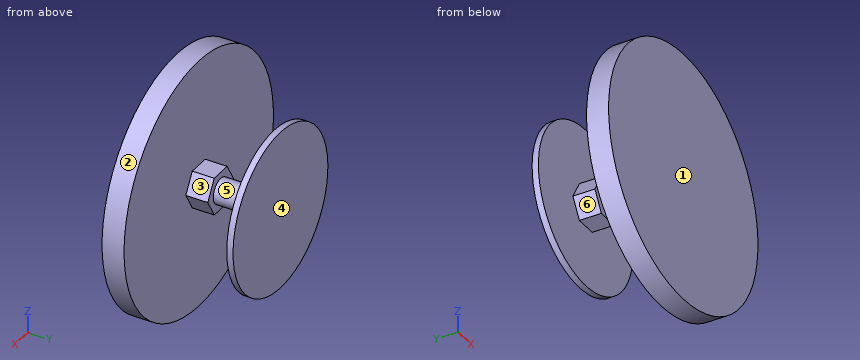
from build123d import *

# Parameters (mm, degrees)
ESBO_O2_R                = 40
RESSALTO_EXTRUS_O1_DEPTH = 7
RESSALTO_EXTRUS_O2_DEPTH = 7
ESBO_O4_R                = 4
RESSALTO_EXTRUS_O3_DEPTH = 10
RESSALTO_EXTRUS_O4_DEPTH = 7
ESBO_O6_R                = 25.4
RESSALTO_EXTRUS_O5_DEPTH = 2


with BuildPart() as part:
    # Esboço2 → Ressalto-extrusão1 (new body)
    with BuildSketch(Plane(origin=(0, 0, 0), x_dir=(1, 0, 0), z_dir=(0, 1, 0))):
        with Locations(Location((0, 0, 0), (0, 0, 270))):
            Circle(ESBO_O2_R)
    extrude(amount=RESSALTO_EXTRUS_O1_DEPTH)

    # Esboço3 → Ressalto-extrusão2 (add)
    with BuildSketch(Plane(origin=(0, 7, 0), x_dir=(1, 0, 0), z_dir=(0, 1, 0))):
        Polygon((6.92820323, 0), (3.464101615, 6), (-3.464101615, 6), (-6.92820323, 0), (-3.464101615, -6), (3.464101615, -6), align=None)
    extrude(amount=RESSALTO_EXTRUS_O2_DEPTH)

    # Esboço4 → Ressalto-extrusão3 (add)
    with BuildSketch(Plane(origin=(0, 14, 0), x_dir=(1, 0, 0), z_dir=(0, 1, 0))):
        with Locations(Location((0, 0, 0), (0, 0, 270))):
            Circle(ESBO_O4_R)
    extrude(amount=RESSALTO_EXTRUS_O3_DEPTH)

    # Esboço5 → Ressalto-extrusão4 (add)
    with BuildSketch(Plane(origin=(0, 24, 0), x_dir=(1, 0, 0), z_dir=(0, 1, 0))):
        Polygon((6.92820323, 0), (3.464101615, 6), (-3.464101615, 6), (-6.92820323, 0), (-3.464101615, -6), (3.464101615, -6), align=None)
    extrude(amount=RESSALTO_EXTRUS_O4_DEPTH)

    # Esboço6 → Ressalto-extrusão5 (add)
    with BuildSketch(Plane(origin=(0, 31, 0), x_dir=(1, 0, 0), z_dir=(0, 1, 0))):
        with Locations(Location((0, 0, 0), (0, 0, 270))):
            Circle(ESBO_O6_R)
    extrude(amount=RESSALTO_EXTRUS_O5_DEPTH)


solid = part.part
Read the model definition and answer for the solid it produces. Units are mm, in the model's axes. Face numbers are marked on the shaded views. A direction names the side the tool comes from. Round coordinates to 2 decimals unless told otherwise and drop trailing zeros. Order: outer loops, then holes, each group sorted by start corner. A loop starts at its lowest first (then second) coordinate and runs counter-clockwise, first axis right, second up. Notation, with made-up numbers: (-4, -34) - (53, -34) arc R34 cw to (53, -3) - close; hole circle Ø7 at (-16, 50). An arc over 180 degrees is marked (long way). Use one line per item in the form item = value. Start each with the question number.
(1) Find the intervals of material crossed by line 1 along Y through (x, z) = (-16.5, 18); line 2 along Y through (x, z) = (33.5, 8.5); line 3 along Z through (x, y) = (-2, 20.5), in increasing order. Write a range as from..to.
(2) The part is cut by section D-D (y = 10). Give the vertices of the cut face in (x, z).
(3) For the marked faces 4, 5 and 6, determine the directions among +Z, -Z, +X, -X, +Y, -Y from which every point of the face is accessible in a straight line to the end or side of a thin tool.
(4) Determine the mould class of the marked faces 1, 2 and 3 for opening direction Y: +Y half, -Y half, draft (parallel to the pull), parting line (faces both ways), or undercut.
(5) The part is cut by section A-A (x = 20.5). Give the vertices of the cut face in (y, z).
(6) The part is cut by section B-B (z = -14.5). Give the vertices of the cut face in (x, y).
(7) The part is cut by section C-C (x = 0). Give the vertices of the cut face in (y, z), then the cut area to 3 significant figures.
(8) Flat-ended cylindrical pins translate along their axes: pin 1 Ø2 at (x, y) = (0, 11.5) entering from -Z; pin 2 Ø3.5 at (x, y) = (0.5, 26.5) entering from +Z; pin 3 Ø1 at (y, z) = (3.5, 31.5) entering from -X; pin 4 Ø10 at (y, z) = (25, 22.5) entering from +X. Find the tip coordinate at first contact, or state that the pin passes through.
Checked values:
q1.line_1 = 0..7, 31..33
q1.line_2 = 0..7
q1.line_3 = -3.46..3.46
q2.outline = (-6.93, 0) - (-3.46, -6) - (3.46, -6) - (6.93, 0) - (3.46, 6) - (-3.46, 6) - close
q3.face_4 = +Z, -Z, +X, -X, +Y
q3.face_5 = none
q3.face_6 = -Z, -X
q4.face_1 = -Y half
q4.face_2 = draft
q4.face_3 = undercut
q5.outline = (0, -34.35) - (7, -34.35) - (7, 34.35) - (0, 34.35) - close; (31, -15) - (33, -15) - (33, 15) - (31, 15) - close
q6.outline = (-37.28, 0) - (37.28, 0) - (37.28, 7) - (-37.28, 7) - close; (-20.85, 31) - (20.85, 31) - (20.85, 33) - (-20.85, 33) - close
q7.outline = (0, -40) - (7, -40) - (7, -6) - (14, -6) - (14, -4) - (24, -4) - (24, -6) - (31, -6) - (31, -25.4) - (33, -25.4) - (33, 25.4) - (31, 25.4) - (31, 6) - (24, 6) - (24, 4) - (14, 4) - (14, 6) - (7, 6) - (7, 40) - (0, 40) - close
q7.area = 910 mm^2
q8.pin_1 = -6
q8.pin_2 = 6
q8.pin_3 = -25.28
q8.pin_4 = through
